Input: part model. Units: mm. Frame: model coordinates. Face numbers are marked on the shaded views. A direction names the side the tool comes from. Round coordinates to 2 decimals unless told otherwise and drop trailing zeros. Loops run counter-clockwise (first coordinate to the right, second up) from the corner with the lowest first, then second, coordinate; pieces in that order, holes last. Notation, with made-up numbers: (85, -2.5) - (136, -2.5) arc R20 ccw to (136, 28.5) - close; hole circle Ø3 at (71, -5). An arc over 180 degrees is marked (long way). One line per question, with ' | ' between items. Start each with the question number.
Item 1: Section A-A, the plane y = -2. Return loops of the section in (x, z).
Item 2: Section B-B, the plane z = 40. Return loops of the section in (x, y).
Item 3: First-contact query: pin 1 (2 mm diameter, centred on y = -2, z = 65.5, fed in from -X). Flat tip, straight axial feed; report the tip coordinate or a pass-through.
Item 4: Draft query along X for the marked faces 1, 2 and 3. Return one class per face: pulls with the +X half, pulls with the -X half, needs draft (parallel to the pull), parting line crosses it, or undercut.
Item 5: Set-up query: the marked faces 4 and 5. Return all of +Z, -Z, +X, -X, +Y, -Y with unobstructed straight access to the full face (end or side cutting, diameter ignored); none if empty.
Item 6: Section C-C, the plane x = 71. Return loops of the section in (y, z).
Item 7: Material intervals for line 1 along Z through (x, y) = (66.5, -4.75); line 2 along Z through (x, y) = (65, -1.25); line 3 along X through (y, z) = (-1.25, 69.5), sorted ascending.
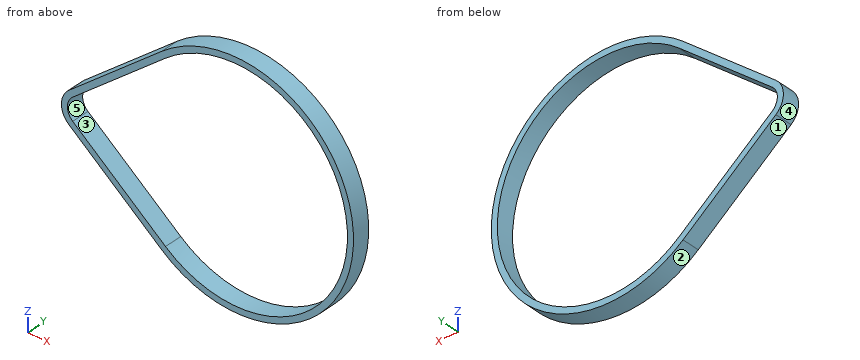
```python
from build123d import *

# Parameters (mm, degrees)
F1_DEPTH = 6
F3_DEPTH = 25
F5_DEPTH = 6


with BuildPart() as f1:
    # F0 (on Front) → F1 (new body)
    with BuildSketch(Plane.XZ):
        with BuildLine():
            Line((58.7550879584, 58.5268499794), (89.4948039231, 33.5402062991))
            ThreePointArc((89.4948039231, 33.5402062991), (151.3819243933, 62.9887506366), (89.4948039231, 92.4372949741))
            Line((89.4948039231, 92.4372949741), (58.7550879584, 67.4506512938))
            ThreePointArc((58.7550879584, 67.4506512938), (56.6319243933, 62.9887506366), (58.7550879584, 58.5268499794))
        make_face()
    extrude(amount=F1_DEPTH)

    # F2 (on face) → F3 (cut)
    with BuildSketch(Plane.XZ.offset(6)):
        with BuildLine():
            Line((90.1255580857, 91.6613122511), (59.385842121, 66.6746685708))
            ThreePointArc((59.385842121, 66.6746685708), (57.6319243933, 62.9887506366), (59.385842121, 59.3028327024))
            Line((59.385842121, 59.3028327024), (90.1255580857, 34.3161890221))
            ThreePointArc((90.1255580857, 34.3161890221), (150.3819243933, 62.9887506366), (90.1255580857, 91.6613122511))
        make_face()
    extrude(amount=-F3_DEPTH, mode=Mode.SUBTRACT)

    # F4 (on face) → F5 (join)
    with BuildSketch(Plane.XZ.offset(6)):
        with BuildLine():
            Line((88.8640497606, 93.2132776971), (58.1243337958, 68.2266340168))
            ThreePointArc((58.1243337958, 68.2266340168), (55.6319243933, 62.9887506366), (58.1243337958, 57.7508672564))
            Line((58.1243337958, 57.7508672564), (88.8640497606, 32.7642235761))
            ThreePointArc((88.8640497606, 32.7642235761), (152.3819243933, 62.9887506366), (88.8640497606, 93.2132776971))
        make_face()
        with BuildLine():
            Line((58.7550879584, 67.4506512938), (89.4948039231, 92.4372949741))
            ThreePointArc((89.4948039231, 92.4372949741), (151.3819243933, 62.9887506366), (89.4948039231, 33.5402062991))
            Line((89.4948039231, 33.5402062991), (58.7550879584, 58.5268499794))
            ThreePointArc((58.7550879584, 58.5268499794), (56.6319243933, 62.9887506366), (58.7550879584, 67.4506512938))
        make_face(mode=Mode.SUBTRACT)
    extrude(amount=-F5_DEPTH)


solid = f1.part
```
Return value:
1) outline: (58.12, 57.75) - (88.86, 32.76) arc R38.95 ccw (long way) to (88.86, 93.21) - (58.12, 68.23) arc R6.75 ccw to start; hole (59.39, 59.3) - (90.13, 34.32) arc R36.95 ccw (long way) to (90.13, 91.66) - (59.39, 66.67) arc R4.75 ccw to start
2) outline: (79.96, -6) - (83.13, -6) - (83.13, 0) - (79.96, 0) - close; (142.36, -6) - (144.87, -6) - (144.87, 0) - (142.36, 0) - close
3) pin 1: x = 55.8
4) face 1: pulls with the -X half | face 2: parting line crosses it | face 3: undercut
5) face 4: -X, +Y, -Y | face 5: +Y, -Y
6) outline: (-6, 47.28) - (0, 47.28) - (0, 49.86) - (-6, 49.86) - close; (-6, 76.12) - (0, 76.12) - (0, 78.69) - (-6, 78.69) - close
7) line 1: 50.94 to 53.52, 72.46 to 75.03 | line 2: 52.16 to 54.74, 71.24 to 73.82 | line 3: 59.69 to 62.86, 149.8 to 151.83
